Could you check a few things on this drawing? It's one solid part, dimensions in mm from its lowest x, y, z. A direction names the side the tool comes from. Round coordinates to 2 decimals unless told otherwise and drop trailing zeros. Write each loop counter-clockwise with the first axis right and the second up, starting at its lowest first coordinate (ties: lowest second). Pieces come first, ordered by that corner, then holes. Notation, with made-up numbers: (-25, 86.25) -> (7, 86.25) arc R28 ccw to (7, 114.25) -> close; hole circle Ø5 at (58, -9.75). An arc over 180 degrees is marked (long way). Answer as CSV lines item,"result".
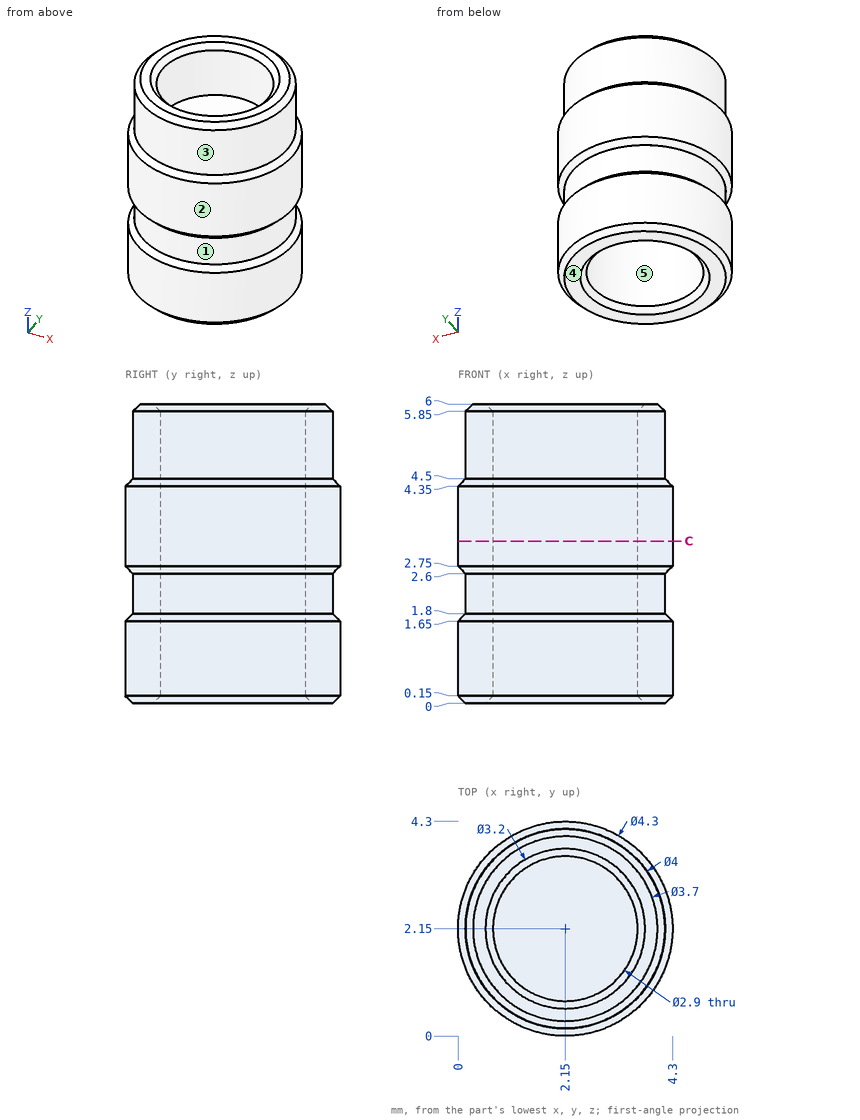
1. If we mould it in two halves opening along Y, with no side actions, what happens to the marked faces 3, 4 and 5? For each: released by +Y, released by -Y, zero draft, split by the parting line, or undercut.
Numbers:
face 3,"split by the parting line"
face 4,"zero draft"
face 5,"undercut"
2. On a 3-axis mill with a long thin cutter (end or side, diameter ignored), from which of +Z, -Z, +X, -X, +Y, -Y can I reach the whole of each face in a straight line? I mean the marked faces 1 and 2. Say none if no direction works.
Numbers:
face 1,"none"
face 2,"+Z, -Z"
3. Suppose I cut it at C-C on z = 3.25. Please give me the cut outline in (x, y).
Numbers:
outline,"circle Ø4.3 at (2.15, 2.15); hole circle Ø2.9 at (2.15, 2.15)"
4. If I drill on line 1 (Y direction, x = 2.15, z = 1.35); line 2 (X direction, y = 2.2, z = 4.8), over which ranges is the centre line in solid material (lowest first)?
Numbers:
line 1,"y = 0 to 0.7, 3.6 to 4.3"
line 2,"x = 0.15 to 0.7, 3.6 to 4.15"
